For this review, take the finished solid that the model builds, in its own axes (mm). A direction names the side the tool comes from. Coordinates: 2 decimals unless noted, no trailing zeros. Write each loop counter-clockwise with the first axis right and the second up, starting at its lowest first coordinate (ties: lowest second). Pieces come first, ordered by that corner, then holes. Notation, with made-up numbers: M -33,51 L -15,51 A9 cw -15,61 Z; hole C 52.25,1 d7. An arc over 180 degrees is marked long. Return JSON: item names as keys, results as strings.
```python
from build123d import *

# Parameters (mm, degrees)
SALIENTE_EXTRUIR1_DEPTH              = 90
CORTAR_EXTRUIR1_DEPTH                = 153.015667403
CORTAR_EXTRUIR1_DEPTH_BACK           = 153.015667403
CROQUIS2_OUTSIDE_W                   = 195.144
CROQUIS2_OUTSIDE_H                   = 235.144
REDONDEO1_R                          = 10
CROQUIS3_R                           = 12
SALIENTE_EXTRUIR2_DEPTH              = 14
CORTAR_EXTRUIR2_DEPTH                = 16
TALADRO1_D                           = 6
TALADRO1_DEPTH                       = 6
TALADRO_ROSCADO_M163_REACH           = 216.283
TALADRO_ROSCADO_M163_BORE_R          = 7
TALADRO_ROSCADO_M163_ON_FACE_2_REACH = 223.31
TALADRO_ROSCADO_M163_BORE_2_R        = 7


with BuildPart() as part:
    # Croquis1 → Saliente-Extruir1 (new, symmetric)
    with BuildSketch(Plane.XY):
        Polygon((-70, -35.859640122), (70, -35.859640122), (70, -19.859640122), (-55.587324838, -19.859640122), (-37.178438023, 84.54234499), (-8.604032122, 84.54234499), (-8.604032122, 100.54234499), (-50.604032122, 100.54234499), (-70, -9.45765501), align=None)
    extrude(amount=SALIENTE_EXTRUIR1_DEPTH, both=True)

    # Croquis2 outside → Cortar-Extruir1 (cut, two sides: drawn at the far end of the back side and taken through both)
    with BuildSketch(Plane(origin=(0, 0, 0), x_dir=(1, 0, 0), z_dir=(0, 1, 0)).offset(-CORTAR_EXTRUIR1_DEPTH_BACK)):
        Rectangle(CROQUIS2_OUTSIDE_W, CROQUIS2_OUTSIDE_H)
        with BuildLine():
            Line((-70, 50), (-70, -50))
            Line((-70, -50), (43.366457067, -82.390416305))
            ThreePointArc((43.366457067, -82.390416305), (61.688422944, -78.981093081), (70, -62.300697244))
            Line((70, -62.300697244), (70, 60.679009052))
            ThreePointArc((70, 60.679009052), (61.20181191, 78.335978242), (41.807165035, 81.944904296))
            Line((41.807165035, 81.944904296), (-70, 50))
        make_face(mode=Mode.SUBTRACT)
    extrude(amount=CORTAR_EXTRUIR1_DEPTH + CORTAR_EXTRUIR1_DEPTH_BACK, mode=Mode.SUBTRACT)

    # Redondeo1
    redondeo1_edges = [part.edges().sort_by_distance(p)[0] for p in [
        (-8.604032122, 92.54234499, -67.541705108),
        (-8.604032122, 92.54234499, 67.541705108),
    ]]
    fillet(redondeo1_edges, radius=REDONDEO1_R)

    # Croquis3 → Saliente-Extruir2 (add)
    with BuildSketch(Plane(origin=(0, -19.859640122, 0), x_dir=(1, 0, 0), z_dir=(0, 1, 0))):
        with Locations((47.883135105, 60.679009052)):
            Circle(CROQUIS3_R)
    saliente_extruir2 = extrude(amount=SALIENTE_EXTRUIR2_DEPTH)

    # Simetría4: Saliente-Extruir2 across plane
    add(saliente_extruir2.mirror(Plane.XY))

    # Croquis4 → Cortar-Extruir2 (cut)
    with BuildSketch(Plane(origin=(0, 100.54234499, 0), x_dir=(1, 0, 0), z_dir=(0, 1, 0))):
        with BuildLine():
            Line((-8.604032122, 25), (-8.604032122, -25))
            ThreePointArc((-8.604032122, -25), (-33.604032122, 0), (-8.604032122, 25))
        make_face()
    extrude(amount=-CORTAR_EXTRUIR2_DEPTH, mode=Mode.SUBTRACT)

    # Croquis5 → Revolución1 (revolve)
    with BuildSketch(Plane.XY, mode=Mode.PRIVATE) as revoluci_n1_sk:
        Polygon((37, 26.140359878), (37, 20.140359878), (26.171234463, 20.140359878), (38, -19.859640122), (33.828765537, -19.859640122), (22, 20.140359878), (22, 26.140359878), align=None)
    revolve(revoluci_n1_sk.sketch.rotate(Axis((2, -40.2659066, 0), (0, 1, 0)), 90), axis=Axis((2, -40.2659066, 0), (0, 1, 0)))

    # Taladro1
    with Locations(Plane(origin=(2, 26.140359878, -27.498672592), x_dir=(0, 0, 1), z_dir=(0, 1, 0))):
        with Locations((0, 0), (27.498673581, 27.497904202), (54.996574558, 0), (27.498672592, -27.501922028)):
            Hole(TALADRO1_D / 2, depth=TALADRO1_DEPTH)

    # Taladro roscado M163 bore (on position points) → Taladro roscado M163 (cut, up to next)
    with BuildSketch(Plane(origin=(47.883135105, -5.859640122, -60.679009052), x_dir=(1, 0, 0), z_dir=(0, 1, 0)), mode=Mode.PRIVATE) as taladro_roscado_m163_sk1:
        Circle(TALADRO_ROSCADO_M163_BORE_R)
    taladro_roscado_m163_tool1 = extrude(taladro_roscado_m163_sk1.sketch, amount=-TALADRO_ROSCADO_M163_REACH, mode=Mode.PRIVATE) & part.part
    add(taladro_roscado_m163_tool1.solids().sort_by_distance((47.883135, -5.85964, -60.679009))[0], mode=Mode.SUBTRACT)

    # Taladro roscado M163 bore 2 (on position points) → Taladro roscado M163 on face 2 (cut, up to next)
    with BuildSketch(Plane(origin=(47.883135105, -19.859640122, 60.679009052), x_dir=(1, 0, 0), z_dir=(0, 1, 0)), mode=Mode.PRIVATE) as taladro_roscado_m163_on_face_2_sk1:
        Circle(TALADRO_ROSCADO_M163_BORE_2_R)
    taladro_roscado_m163_on_face_2_tool1 = extrude(taladro_roscado_m163_on_face_2_sk1.sketch, amount=-TALADRO_ROSCADO_M163_ON_FACE_2_REACH, mode=Mode.PRIVATE) & part.part
    add(taladro_roscado_m163_on_face_2_tool1.solids().sort_by_distance((47.883135, -19.85964, 60.679009))[0], mode=Mode.SUBTRACT)


solid = part.part
```
1. Wall thickness on L1, parallel to Y at x = -29, z = -26.5; L2, parallel to X at y = 24.25, z = 0; L3, parallel to Y at x = 15, z = -47: over which ranges is each line inside the solid? List them lowest first. Write a range as from..to.
Checks:
{"L1": "-35.86..-19.86, 84.54..100.54", "L2": "-64.06..-47.81, -33..-28.5, -22.5..-18, 22..26.5, 32.5..37", "L3": "-35.86..-19.86"}
2. Draft analysis for pull direction Z (two halves, no side actions). For faces 1 (the face through (17, 26.14, 15)), 2 (the face through (-51.1, 11.8, -55.4)), 3 (the face through (2.1, 23.1, -24.5)), state which applies: +Z half, -Z half, draft (parallel to the pull), parting line (faces both ways), or undercut.
Checks:
{"face 1": "draft", "face 2": "-Z half", "face 3": "undercut"}
3. We need section B-B (x = -47). State the section outline as (y, z) points.
Checks:
{"outline": "M -35.86,-56.57 L -19.86,-56.57 L -19.86,56.57 L -35.86,56.57 Z; M 28.84,-56.57 L 100.54,-56.57 L 100.54,56.57 L 28.84,56.57 Z"}
4. We need section D-D (x = 2). State the section outline as (y, z) points.
Checks:
{"outline": "M -35.86,-70.57 L -19.86,-70.57 L -19.86,-36 L 20.14,-24.17 L 20.14,-24.5 L 26.14,-24.5 L 26.14,-20 L 20.14,-20 L -19.86,-31.83 L -19.86,31.83 L 20.14,20 L 26.14,20 L 26.14,24.5 L 20.14,24.5 L 20.14,24.17 L -19.86,36 L -19.86,70.57 L -35.86,70.57 Z; M 20.14,-35 L 26.14,-35 L 26.14,-30.5 L 20.14,-30.5 Z; M 20.14,30.5 L 26.14,30.5 L 26.14,35 L 20.14,35 Z"}
5. We need section C-C (z = 0). Give the number of separate pieces and of enclosed holes in the cut face, plus the area to 3 significant figures.
Checks:
{"separate pieces": "3", "enclosed holes": "0", "area": "4,660 mm2"}
6. Clearance check with flat-ended pins moving along their axes: pin 1 Ø7 at (x, z) = (46.5, 60.5) entering from -Y; pin 2 Ø7 at (x, z) = (53.5, -58.5) entering from +Y; pin 3 Ø3 at (y, z) = (73, -38) entering from +X. State where each tip first meets the part, or that it passes through.
Checks:
{"pin 1": "y = -19.86", "pin 2": "y = -5.86", "pin 3": "x = -38.95"}
7. For faces 4 (the face through (51.11, -27.75, 66.89)), 5 (the face through (14, 23, 16)), 6 (the face through (25, 20.14, 8)), list the 3-axis set-ups (+Z, -Z, +X, -X, +Y, -Y) from which the entire face can be reached by the end or side of a thin tool; tool diameter is ignored.
Checks:
{"face 4": "-Y", "face 5": "+Y", "face 6": "none"}
8. We need section A-A (y = 4). State the section outline as (x, z) points.
Checks:
{"outline": "M -67.63,-50.68 L -51.38,-55.32 L -51.38,55.32 L -67.63,50.68 Z; C 2,0 d57.89; hole C 2,0 d49.55"}
